from build123d import *

# Parameters (mm, degrees)
F0_W     = 15
F0_H     = 28
F0_R     = 1.8
F0_R_2   = 5.5
F0_R_3   = 4
F1_DEPTH = 5
F2_DEPTH = 15


with BuildPart() as f1:
    # F0 (on Front) → F1 (new body)
    with BuildSketch(Plane.XZ):
        Rectangle(F0_W, F0_H)
        with Locations((0, -10)):
            Circle(F0_R, mode=Mode.SUBTRACT)
        with Locations((0, -4)):
            Circle(F0_R, mode=Mode.SUBTRACT)
        with Locations((0, 8)):
            Circle(F0_R_2, mode=Mode.SUBTRACT)
        with Locations((0, 8)):
            Circle(F0_R_2)
        with Locations((0, 8)):
            Circle(F0_R_3, mode=Mode.SUBTRACT)
        with Locations((0, 8)):
            Circle(F0_R_3)
    extrude(amount=-F1_DEPTH)

    # F0 (on Front) → F2 (join)
    with BuildSketch(Plane.XZ):
        with Locations((0, 8)):
            Circle(F0_R_2)
        with Locations((0, 8)):
            Circle(F0_R_3, mode=Mode.SUBTRACT)
    extrude(amount=F2_DEPTH)


solid = f1.part
The model under review builds one solid part; all positions refer to its coordinate system, in mm. A direction names the side the tool comes from. Coordinates: 2 decimals unless noted, no trailing zeros. Write each loop counter-clockwise with the first axis right and the second up, starting at its lowest first coordinate (ties: lowest second). Pieces come first, ordered by that corner, then holes. Notation, with made-up numbers: M 36,-33 L 93,-33 A32 ccw 93,-7 Z; hole C 49.5,24 d10. An arc over 180 degrees is marked long. Put each result on its own line as item: value.
1) Draft analysis for pull direction Z (two halves, no side actions). For faces 1 (the flat face through (0, 5, 0)), 2 (the cylindrical face through (-0.234, 2.465, -2.215)), 3 (the flat face through (0, 2, 14)), state which applies: released by +Z, released by -Z, zero draft, split by the parting line, or undercut.
Computed:
face 1: zero draft
face 2: undercut
face 3: released by +Z
2) Wall thickness on probe 1 along Z at (x, y) = (0, 2.95); probe 2 along Z at (x, y) = (1, 1); probe 3 along Y at (x, z) = (-5, 12.75): over which ranges is each line inside the solid? List them lowest first. Write a range as [from, to].
Computed:
probe 1: z = [-14, -11.8], [-8.2, -5.8], [-2.2, 14]
probe 2: z = [-14, -11.5], [-8.5, -5.5], [-2.5, 14]
probe 3: y = [0, 5]
3) Add section D-D on z = 8. Give the boundary of the cut face in (x, y), then the cut area to 3 significant figures.
Computed:
outline: M -7.5,0 L -5.5,0 L -5.5,-15 L -4,-15 L -4,0 L 4,0 L 4,-15 L 5.5,-15 L 5.5,0 L 7.5,0 L 7.5,5 L -7.5,5 Z
area: 120 mm2
4) Add section B-B on z = -4. Give the boundary of the cut face in (x, y), then the cut area to 3 significant figures.
Computed:
outline: M -7.5,0 L -1.8,0 L -1.8,5 L -7.5,5 Z; M 1.8,0 L 7.5,0 L 7.5,5 L 1.8,5 Z
area: 57.0 mm2
5) Add section C-C on y = 0.5. Give the boundary of the cut face in (x, z).
Computed:
outline: M -7.5,-14 L 7.5,-14 L 7.5,14 L -7.5,14 Z; hole C 0,-10 d3.6; hole C 0,-4 d3.6
6) Add section A-A on x = 0. Give the boundary of the cut face in (y, z).
Computed:
outline: M -15,2.5 L 0,2.5 L 0,-2.2 L 5,-2.2 L 5,14 L 0,14 L 0,13.5 L -15,13.5 L -15,12 L 0,12 L 0,4 L -15,4 Z; M 0,-14 L 5,-14 L 5,-11.8 L 0,-11.8 Z; M 0,-8.2 L 5,-8.2 L 5,-5.8 L 0,-5.8 Z
7) For faces 4 (the flat face through (0, 0, 8)), 5 (the flat face through (7.5, 2, 0)), list the 3-axis set-ups (+Z, -Z, +X, -X, +Y, -Y) from which the entire face can be reached by the end or side of a thin tool; tool diameter is ignored.
Computed:
face 4: -Y
face 5: +Z, -Z, +X, +Y, -Y
8) Clearance check with flat-ended pins moving along their axes: pin 1 Ø1.5 at (x, z) = (-5.5, -3) entering from -Y; pin 2 Ø3 at (x, z) = (0, -10) entering from -Y; pin 3 Ø3 at (x, y) = (-2.5, -9.5) entering from +Z; pin 4 Ø5 at (x, y) = (2.5, -5) entering from -Z. State where each tip first meets the part, or that it passes through.
Computed:
pin 1: stops at y = 0
pin 2: passes through
pin 3: stops at z = 13.41
pin 4: stops at z = 2.5
